```python
from build123d import *

# Parameters (mm, degrees)
BOSS_EXTRUDE2_DEPTH  = 2
SKETCH3_W            = 6
SKETCH3_H            = 6
CUT_EXTRUDE1_DEPTH   = 2
SKETCH4_R            = 5
BOSS_EXTRUDE3_DEPTH  = 1.5
SKETCH5_W            = 12
SKETCH5_H            = 12
BOSS_EXTRUDE4_DEPTH  = 1
SKETCH6_W            = 6
SKETCH6_H            = 6
CUT_EXTRUDE2_DEPTH   = 10
SKETCH7_W            = 16
SKETCH7_H            = 16
BOSS_EXTRUDE5_DEPTH  = 1
SKETCH9_R            = 6
BOSS_EXTRUDE6_DEPTH  = 1
SKETCH10_W           = 6
SKETCH10_H           = 6
CUT_EXTRUDE3_DEPTH   = 10
BOSS_EXTRUDE7_DEPTH  = 3
CUT_EXTRUDE4_DEPTH   = 1
SKETCH13_W           = 14
SKETCH13_H           = 14
SKETCH13_W_2         = 10
SKETCH13_H_2         = 10
CUT_EXTRUDE5_DEPTH   = 1.5
BOSS_EXTRUDE8_DEPTH  = 3
SKETCH16_R           = 7
BOSS_EXTRUDE9_DEPTH  = 1
SKETCH17_W           = 6
SKETCH17_H           = 6
CUT_EXTRUDE7_DEPTH   = 4
SKETCH18_W           = 8
SKETCH18_H           = 8
CUT_EXTRUDE8_DEPTH   = 10
SKETCH19_W           = 12
SKETCH19_H           = 12
SKETCH19_W_2         = 8
SKETCH19_H_2         = 8
BOSS_EXTRUDE10_DEPTH = 1.5
SKETCH20_W           = 16
SKETCH20_H           = 16
SKETCH20_W_2         = 12
SKETCH20_H_2         = 12
CUT_EXTRUDE9_DEPTH   = 1.5
SKETCH23_W           = 10
SKETCH23_H           = 10
SKETCH23_W_2         = 8
SKETCH23_H_2         = 8
CUT_EXTRUDE15_DEPTH  = 10
SKETCH24_R           = 8
BOSS_EXTRUDE11_DEPTH = 1
SKETCH25_W           = 10
SKETCH25_H           = 10
CUT_EXTRUDE16_DEPTH  = 1
BOSS_EXTRUDE12_DEPTH = 1
SKETCH27_W           = 10
SKETCH27_H           = 10
CUT_EXTRUDE17_DEPTH  = 1
SKETCH28_W           = 14
SKETCH28_H           = 14
SKETCH28_W_2         = 12
SKETCH28_H_2         = 12
BOSS_EXTRUDE13_DEPTH = 1.5
SKETCH29_W           = 18
SKETCH29_H           = 18
SKETCH29_W_2         = 16
SKETCH29_H_2         = 16
CUT_EXTRUDE18_DEPTH  = 1.5
BOSS_EXTRUDE14_START = 0.2
BOSS_EXTRUDE14_DEPTH = 0.2
SKETCH31_R           = 2
CUT_EXTRUDE19_DEPTH  = 7.826


with BuildPart() as part:
    # Sketch2 → Boss-Extrude2 (new body)
    with BuildSketch(Plane(origin=(0, 0, 0), x_dir=(0, 0, -1), z_dir=(1, 0, 0))):
        with BuildLine():
            Line((2.54, 0), (27.46, 0))
            ThreePointArc((27.46, 0), (29.256051224, 0.743948776), (30, 2.54))
            Line((30, 2.54), (30, 37.46))
            ThreePointArc((30, 37.46), (29.256051224, 39.256051224), (27.46, 40))
            Line((27.46, 40), (2.54, 40))
            ThreePointArc((2.54, 40), (0.743948776, 39.256051224), (0, 37.46))
            Line((0, 37.46), (0, 2.54))
            ThreePointArc((0, 2.54), (0.743948776, 0.743948776), (2.54, 0))
        make_face()
    extrude(amount=BOSS_EXTRUDE2_DEPTH)

    # Sketch3 → Cut-Extrude1 (cut)
    with BuildSketch(Plane.ZY):
        with Locations((-15, 20)):
            Rectangle(SKETCH3_W, SKETCH3_H)
    extrude(amount=-CUT_EXTRUDE1_DEPTH, mode=Mode.SUBTRACT)

    # Sketch4 → Boss-Extrude3 (add)
    with BuildSketch(Plane.ZY):
        with Locations((-15, 20)):
            Circle(SKETCH4_R)
    extrude(amount=BOSS_EXTRUDE3_DEPTH)

    # Sketch5 → Boss-Extrude4 (add)
    with BuildSketch(Plane.ZY):
        with Locations((-15, 20)):
            Rectangle(SKETCH5_W, SKETCH5_H)
    extrude(amount=BOSS_EXTRUDE4_DEPTH)

    # Sketch6 → Cut-Extrude2 (cut)
    with BuildSketch(Plane(origin=(2, 0, 0), x_dir=(0, 0, -1), z_dir=(1, 0, 0))):
        with Locations((15, 20)):
            Rectangle(SKETCH6_W, SKETCH6_H)
    extrude(amount=-CUT_EXTRUDE2_DEPTH, mode=Mode.SUBTRACT)

    # Sketch7 → Boss-Extrude5 (add)
    with BuildSketch(Plane.ZY):
        with Locations((-15, 20)):
            Rectangle(SKETCH7_W, SKETCH7_H)
    extrude(amount=BOSS_EXTRUDE5_DEPTH)

    # Sketch9 → Boss-Extrude6 (add)
    with BuildSketch(Plane.ZY.offset(1)):
        with Locations(Location((-15, 20, 0), (0, 0, 180))):
            Circle(SKETCH9_R)
    extrude(amount=BOSS_EXTRUDE6_DEPTH)

    # Sketch10 → Cut-Extrude3 (cut)
    with BuildSketch(Plane(origin=(0, 0, 0), x_dir=(0, 0, -1), z_dir=(1, 0, 0))):
        with Locations((15, 20)):
            Rectangle(SKETCH10_W, SKETCH10_H)
    extrude(amount=-CUT_EXTRUDE3_DEPTH, mode=Mode.SUBTRACT)

    # Sketch11 → Boss-Extrude7 (add)
    with BuildSketch(Plane(origin=(2, 0, 0), x_dir=(0, 0, -1), z_dir=(1, 0, 0))):
        with BuildLine():
            Line((4.54, 38), (25.46, 38))
            ThreePointArc((25.46, 38), (27.256051224, 37.256051224), (28, 35.46))
            Line((28, 35.46), (28, 4.54))
            ThreePointArc((28, 4.54), (27.256051224, 2.743948776), (25.46, 2))
            Line((25.46, 2), (4.54, 2))
            ThreePointArc((4.54, 2), (2.743948776, 2.743948776), (2, 4.54))
            Line((2, 4.54), (2, 35.46))
            ThreePointArc((2, 35.46), (2.743948776, 37.256051224), (4.54, 38))
        make_face()
        with BuildLine():
            Line((6.54, 36), (23.46, 36))
            ThreePointArc((23.46, 36), (25.256051224, 35.256051224), (26, 33.46))
            Line((26, 33.46), (26, 6.54))
            ThreePointArc((26, 6.54), (25.256051224, 4.743948776), (23.46, 4))
            Line((23.46, 4), (6.54, 4))
            ThreePointArc((6.54, 4), (4.743948776, 4.743948776), (4, 6.54))
            Line((4, 6.54), (4, 33.46))
            ThreePointArc((4, 33.46), (4.743948776, 35.256051224), (6.54, 36))
        make_face(mode=Mode.SUBTRACT)
    extrude(amount=BOSS_EXTRUDE7_DEPTH)

    # Sketch12 → Cut-Extrude4 (cut)
    with BuildSketch(Plane.ZY.offset(1)):
        with BuildLine():
            Line((-23, 28), (-20.46, 28))
            ThreePointArc((-20.46, 28), (-22.256051224, 27.256051224), (-23, 25.46))
            Line((-23, 25.46), (-23, 28))
        make_face()
        with BuildLine():
            Line((-7, 28), (-7, 25.46))
            ThreePointArc((-7, 25.46), (-7.743948776, 27.256051224), (-9.54, 28))
            Line((-9.54, 28), (-7, 28))
        make_face()
        with BuildLine():
            Line((-7, 12), (-9.54, 12))
            ThreePointArc((-9.54, 12), (-7.743948776, 12.743948776), (-7, 14.54))
            Line((-7, 14.54), (-7, 12))
        make_face()
        with BuildLine():
            Line((-23, 12), (-23, 14.54))
            ThreePointArc((-23, 14.54), (-22.256051224, 12.743948776), (-20.46, 12))
            Line((-20.46, 12), (-23, 12))
        make_face()
    extrude(amount=-CUT_EXTRUDE4_DEPTH, mode=Mode.SUBTRACT)

    # Sketch13 → Cut-Extrude5 (cut)
    with BuildSketch(Plane(origin=(2, 0, 0), x_dir=(0, 0, -1), z_dir=(1, 0, 0))):
        with Locations((15, 20)):
            Rectangle(SKETCH13_W, SKETCH13_H)
        with Locations((15, 20)):
            Rectangle(SKETCH13_W_2, SKETCH13_H_2, mode=Mode.SUBTRACT)
    extrude(amount=-CUT_EXTRUDE5_DEPTH, mode=Mode.SUBTRACT)

    # Sketch14 → Boss-Extrude8 (add)
    with BuildSketch(Plane.ZY.offset(2)):
        with BuildLine():
            Line((-17.46, 25), (-12.54, 25))
            ThreePointArc((-12.54, 25), (-10.743948776, 24.256051224), (-10, 22.46))
            Line((-10, 22.46), (-10, 17.54))
            ThreePointArc((-10, 17.54), (-10.743948776, 15.743948776), (-12.54, 15))
            Line((-12.54, 15), (-17.46, 15))
            ThreePointArc((-17.46, 15), (-19.256051224, 15.743948776), (-20, 17.54))
            Line((-20, 17.54), (-20, 22.46))
            ThreePointArc((-20, 22.46), (-19.256051224, 24.256051224), (-17.46, 25))
        make_face()
    extrude(amount=-BOSS_EXTRUDE8_DEPTH)

    # Sketch16 → Boss-Extrude9 (add)
    with BuildSketch(Plane.ZY.offset(2)):
        with Locations((-15, 20)):
            Circle(SKETCH16_R)
    extrude(amount=-BOSS_EXTRUDE9_DEPTH)

    # Sketch17 → Cut-Extrude7 (cut)
    with BuildSketch(Plane(origin=(1, 0, 0), x_dir=(0, 0, -1), z_dir=(1, 0, 0))):
        with Locations((15, 20)):
            Rectangle(SKETCH17_W, SKETCH17_H)
    extrude(amount=-CUT_EXTRUDE7_DEPTH, mode=Mode.SUBTRACT)

    # Sketch18 → Cut-Extrude8 (cut)
    with BuildSketch(Plane.ZY.offset(2)):
        with Locations((-15, 20)):
            Rectangle(SKETCH18_W, SKETCH18_H)
    extrude(amount=-CUT_EXTRUDE8_DEPTH, mode=Mode.SUBTRACT)

    # Sketch19 → Boss-Extrude10 (add)
    with BuildSketch(Plane(origin=(0.5, 0, 0), x_dir=(0, 0, -1), z_dir=(1, 0, 0))):
        with Locations((15, 20)):
            Rectangle(SKETCH19_W, SKETCH19_H)
        with Locations((15, 20)):
            Rectangle(SKETCH19_W_2, SKETCH19_H_2, mode=Mode.SUBTRACT)
    extrude(amount=BOSS_EXTRUDE10_DEPTH)

    # Sketch20 → Cut-Extrude9 (cut)
    with BuildSketch(Plane(origin=(2, 0, 0), x_dir=(0, 0, -1), z_dir=(1, 0, 0))):
        with Locations((15, 20)):
            Rectangle(SKETCH20_W, SKETCH20_H)
        with Locations((15, 20)):
            Rectangle(SKETCH20_W_2, SKETCH20_H_2, mode=Mode.SUBTRACT)
    extrude(amount=-CUT_EXTRUDE9_DEPTH, mode=Mode.SUBTRACT)

    # Sketch23 → Cut-Extrude15 (cut)
    with BuildSketch(Plane(origin=(2, 0, 0), x_dir=(0, 0, -1), z_dir=(1, 0, 0))):
        with Locations((15, 20)):
            Rectangle(SKETCH23_W, SKETCH23_H)
        with Locations((15, 20)):
            Rectangle(SKETCH23_W_2, SKETCH23_H_2, mode=Mode.SUBTRACT)
    extrude(amount=-CUT_EXTRUDE15_DEPTH, mode=Mode.SUBTRACT)

    # Sketch24 → Boss-Extrude11 (add)
    with BuildSketch(Plane.ZY.offset(1)):
        with Locations((-15, 20)):
            Circle(SKETCH24_R)
    extrude(amount=BOSS_EXTRUDE11_DEPTH)

    # Sketch25 → Cut-Extrude16 (cut)
    with BuildSketch(Plane(origin=(-1, 0, 0), x_dir=(0, 0, -1), z_dir=(1, 0, 0))):
        with Locations((15, 20)):
            Rectangle(SKETCH25_W, SKETCH25_H)
    extrude(amount=-CUT_EXTRUDE16_DEPTH, mode=Mode.SUBTRACT)

    # Sketch26 → Boss-Extrude12 (add)
    with BuildSketch(Plane.ZY):
        with BuildLine():
            Line((-21.46, 29), (-8.54, 29))
            ThreePointArc((-8.54, 29), (-6.743948776, 28.256051224), (-6, 26.46))
            Line((-6, 26.46), (-6, 13.54))
            ThreePointArc((-6, 13.54), (-6.743948776, 11.743948776), (-8.54, 11))
            Line((-8.54, 11), (-21.46, 11))
            ThreePointArc((-21.46, 11), (-23.256051224, 11.743948776), (-24, 13.54))
            Line((-24, 13.54), (-24, 26.46))
            ThreePointArc((-24, 26.46), (-23.256051224, 28.256051224), (-21.46, 29))
        make_face()
    extrude(amount=BOSS_EXTRUDE12_DEPTH)

    # Sketch27 → Cut-Extrude17 (cut)
    with BuildSketch(Plane(origin=(0, 0, 0), x_dir=(0, 0, -1), z_dir=(1, 0, 0))):
        with Locations((15, 20)):
            Rectangle(SKETCH27_W, SKETCH27_H)
    extrude(amount=-CUT_EXTRUDE17_DEPTH, mode=Mode.SUBTRACT)

    # Sketch28 → Boss-Extrude13 (add)
    with BuildSketch(Plane(origin=(0.5, 0, 0), x_dir=(0, 0, -1), z_dir=(1, 0, 0))):
        with Locations((15, 20)):
            Rectangle(SKETCH28_W, SKETCH28_H)
        with Locations((15, 20)):
            Rectangle(SKETCH28_W_2, SKETCH28_H_2, mode=Mode.SUBTRACT)
    extrude(amount=BOSS_EXTRUDE13_DEPTH)

    # Sketch29 → Cut-Extrude18 (cut)
    with BuildSketch(Plane(origin=(2, 0, 0), x_dir=(0, 0, -1), z_dir=(1, 0, 0))):
        with Locations((15, 20)):
            Rectangle(SKETCH29_W, SKETCH29_H)
        with Locations((15, 20)):
            Rectangle(SKETCH29_W_2, SKETCH29_H_2, mode=Mode.SUBTRACT)
    extrude(amount=-CUT_EXTRUDE18_DEPTH, mode=Mode.SUBTRACT)

    # Sketch30 → Boss-Extrude14 (add)
    with BuildSketch(Plane.ZY.offset(BOSS_EXTRUDE14_START)):
        with BuildLine():
            Line((-27.46, 40), (-2.54, 40))
            ThreePointArc((-2.54, 40), (-0.743948776, 39.256051224), (0, 37.46))
            Line((0, 37.46), (0, 2.54))
            ThreePointArc((0, 2.54), (-0.743948776, 0.743948776), (-2.54, 0))
            Line((-2.54, 0), (-27.46, 0))
            ThreePointArc((-27.46, 0), (-29.256051224, 0.743948776), (-30, 2.54))
            Line((-30, 2.54), (-30, 37.46))
            ThreePointArc((-30, 37.46), (-29.256051224, 39.256051224), (-27.46, 40))
        make_face()
        with BuildLine():
            Line((-26.96, 39.5), (-3.04, 39.5))
            ThreePointArc((-3.04, 39.5), (-1.243948776, 38.756051224), (-0.5, 36.96))
            Line((-0.5, 36.96), (-0.5, 3.14))
            ThreePointArc((-0.5, 3.14), (-1.243948776, 1.343948776), (-3.04, 0.6))
            Line((-3.04, 0.6), (-26.96, 0.6))
            ThreePointArc((-26.96, 0.6), (-28.756051224, 1.343948776), (-29.5, 3.14))
            Line((-29.5, 3.14), (-29.5, 36.96))
            ThreePointArc((-29.5, 36.96), (-28.756051224, 38.756051224), (-26.96, 39.5))
        make_face(mode=Mode.SUBTRACT)
    extrude(amount=-BOSS_EXTRUDE14_DEPTH)

    # Sketch31 → Cut-Extrude19 (cut, symmetric)
    with BuildSketch(Plane(origin=(2, 0, 0), x_dir=(0, 0, -1), z_dir=(1, 0, 0))):
        with Locations(Location((5.2, 35, 0), (0, 0, 30))):
            Circle(SKETCH31_R)
        with Locations(Location((24.8, 35, 0), (0, 0, 306.869897646))):
            Circle(SKETCH31_R)
        with Locations(Location((24.8, 5, 0), (0, 0, 53.130102354))):
            Circle(SKETCH31_R)
        with Locations(Location((5.5, 5, 0), (0, 0, 330))):
            Circle(SKETCH31_R)
    extrude(amount=CUT_EXTRUDE19_DEPTH, both=True, mode=Mode.SUBTRACT)


solid = part.part
```
Build history of the part. All positions in model axes, mm. A direction names the side the tool comes from. Coordinates: 2 decimals unless noted, no trailing zeros. Order: outer loops, then holes, each group sorted by start corner. A loop starts at its lowest first (then second) coordinate and runs counter-clockwise, first axis right, second up.
Item 1: Saw through at A-A on z = -24.8. List the corners of the cut face in (x, y), then the cut area to 3 significant figures.
Filled in:
outline: (-0.2, 0) - (2, 0) - (2, 2) - (5, 2) - (5, 3) - (0, 3) - (0, 0.6) - (-0.2, 0.6) - close; (-0.2, 39.5) - (0, 39.5) - (0, 37) - (5, 37) - (5, 38) - (2, 38) - (2, 40) - (-0.2, 40) - close; (0, 7) - (2, 7) - (2, 33) - (0, 33) - close
area: 70.2 mm2
Item 2: Mould opens along Y. For faces 6 (the cylindrical face through (3.479, 37.236, -2.724)), 7 (the flat face through (3, 20, -26)), 8 (the cylindrical face through (3.479, 2.724, -2.764)) say: released by +Y, released by -Y, zero draft, split by the parting line, or undercut.
Filled in:
face 6: released by +Y
face 7: undercut
face 8: released by -Y
Item 3: Drill centre lines: L1, parallel to Y at x = 1, z = -14.75; L2, parallel to Y at x = 1.2, z = -24.8; L3, parallel to Z at x = 2.25, y = 12. Where is each one in solid material? Low to high.
Filled in:
L1: y = 0 to 11, 13 to 15, 25 to 27, 29 to 40
L2: y = 0 to 3, 7 to 33, 37 to 40
L3: z = -28 to -26, -4 to -2
Item 4: Saw through at B-B on y = 35. List the corners of the cut face in (x, z), then the cut area to 3 significant figures.
Filled in:
outline: (-0.2, -30) - (2, -30) - (2, -28) - (5, -28) - (5, -26.8) - (0, -26.8) - (0, -29.5) - (-0.2, -29.5) - close; (-0.2, -0.5) - (0, -0.5) - (0, -3.2) - (5, -3.2) - (5, -2) - (2, -2) - (2, 0) - (-0.2, 0) - close; (0, -22.8) - (2, -22.8) - (2, -7.2) - (0, -7.2) - close
area: 51.4 mm2
Item 5: Drop flat-ended pins along their axis: pin 1 Ø1.5 at (y, z) = (32.5, -16.5) entering from -X; pin 2 Ø17.5 at (y, z) = (15.5, -15.5) entering from +X; pin 3 Ø1.5 at (x, y) = (4, 19) entering from +Z. Give the stop position or say it passes through.
Filled in:
pin 1: stops at x = 0
pin 2: stops at x = 2
pin 3: stops at z = -2
Item 6: Tool access for faces 1 (the flat face through (2, 21.6, -1.6)), 2 (the flat face through (3, 2, -15)), 3 (the flat face through (0, 15, -15)), 4 (the flat face through (3, 20, -28)), 5 (the flat face through (-0.5, 19.9, -24)): list every direction of +Z, -Z, +X, -X, +Y, -Y with a clear straight run to the whole face (end or side of a thin tool).
Filled in:
face 1: +X
face 2: +Z, -Z, +X, -Y
face 3: +X, -X
face 4: -Z, +X, +Y, -Y
face 5: -X
Item 7: Saw through at D-D on y = 12.5. List the corners of the cut face in (x, z), then the cut area to 3 significant figures.
Filled in:
outline: (-2, -17.78) - (-1, -17.78) - (-1, -23.78) - (0, -23.78) - (0, -29.5) - (-0.2, -29.5) - (-0.2, -30) - (2, -30) - (2, -28) - (5, -28) - (5, -26) - (2, -26) - (2, -24) - (0.5, -24) - (0.5, -6) - (2, -6) - (2, -4) - (5, -4) - (5, -2) - (2, -2) - (2, 0) - (-0.2, 0) - (-0.2, -0.5) - (0, -0.5) - (0, -6.22) - (-1, -6.22) - (-1, -12.22) - (-2, -12.22) - close
area: 68.3 mm2
Item 8: Saw through at C-C on x = 4. List the corners of the cut face in (y, z).
Filled in:
outline: (2, -25.46) arc R2.54 ccw to (4.54, -28) - (35.46, -28) arc R2.54 ccw to (38, -25.46) - (38, -4.54) arc R2.54 ccw to (35.46, -2) - (4.54, -2) arc R2.54 ccw to (2, -4.54) - close; hole (4, -23.07) arc R2 ccw (long way) to (6.6, -26) - (33.4, -26) arc R2 ccw (long way) to (36, -23.07) - (36, -6.93) arc R2 ccw (long way) to (33.4, -4) - (6.54, -4) arc R2.54 ccw to (6.33, -4.01) arc R2 ccw (long way) to (4, -7.23) - close
